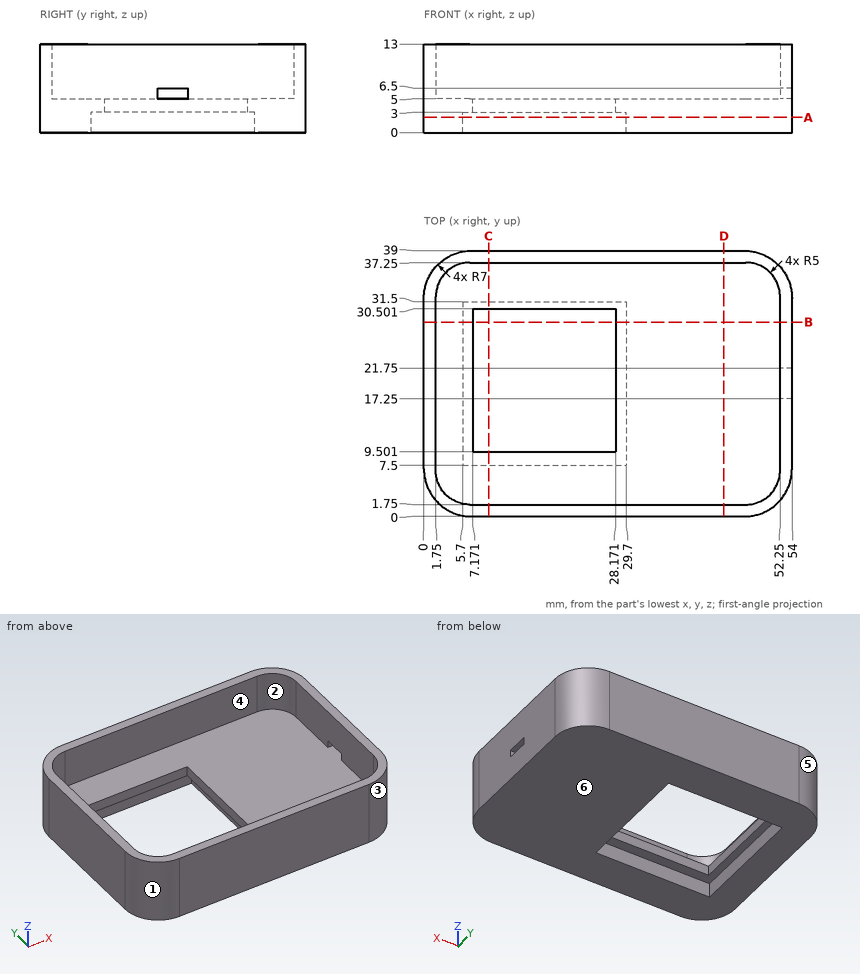
Input: dimensioned drawing with shaded views. Units: mm. Origin: part minimum x, y, z. A direction names the side the tool comes from. Coordinates: 2 decimals unless noted, no trailing zeros. Loops run counter-clockwise (first coordinate to the right, second up) from the corner with the lowest first, then second, coordinate; pieces in that order, holes last. Notation, with made-up numbers: M -25.5,5 L 25.5,5 A23 cw 25.5,26 Z; hole C -34.75,36 d3. An arc over 180 degrees is marked long. Put each result on its own line as item: value.
(1) Cut plane A-A on z = 2.25. Return the cut outline in (x, y), then the cut area to 3 significant figures.
Answer sheet:
outline: M 0,7 A7 ccw 7,0 L 47,0 A7 ccw 54,7 L 54,32 A7 ccw 47,39 L 7,39 A7 ccw 0,32 Z; hole M 5.7,7.5 L 29.7,7.5 L 29.7,31.5 L 5.7,31.5 Z
area: 1,490 mm^2
(2) Access query for the marked faces 1 and 2. Directions: +Z, -Z, +X, -X, +Y, -Y. A direction counts if a zero-diameter tool reaches every point of the face in a straight line with its end or side. Return the directions, or none.
Answer sheet:
face 1: +Z, -Z, -X, -Y
face 2: +Z
(3) Draft query along X for the marked faces 3, 4, 5 and 6. Return one class per face: pulls with the +X half, pulls with the -X half, needs draft (parallel to the pull), parting line crosses it, or undercut.
Answer sheet:
face 3: pulls with the +X half
face 4: undercut
face 5: pulls with the -X half
face 6: needs draft
(4) First-contact query: pin 1 (3.5 mm diameter, centred on x = 12.5, z = 1.5, fed in from -Y); pin 2 (4 mm diameter, centred on x = 17, y = 29.5, fed in from +Z); pin 3 (1.6 mm diameter, centred on x = 53, z = 6, fed in from +Y); pin 4 (0.8 mm diameter, centred on x = 53, z = 5.5, fed in from -Y). Flat tips, straight axial feed; report the tip coordinate or a pass-through.
Answer sheet:
pin 1: stops at y = 0
pin 2: stops at z = 5
pin 3: stops at y = 36.69
pin 4: stops at y = 2.8
(5) Cut plane D-D on x = 44. Return the cut outline in (y, z).
Answer sheet:
outline: M 0,0 L 39,0 L 39,13 L 37.25,13 L 37.25,5 L 1.75,5 L 1.75,13 L 0,13 Z
(6) Cut plane C-C on x = 9.5. Return the cut outline in (y, z).
Answer sheet:
outline: M 0,0 L 7.5,0 L 7.5,3 L 9.5,3 L 9.5,5 L 1.75,5 L 1.75,13 L 0,13 Z; M 30.5,3 L 31.5,3 L 31.5,0 L 39,0 L 39,13 L 37.25,13 L 37.25,5 L 30.5,5 Z
(7) Material intervals for probe 1 along X at (y, z) = (31, 7); probe 2 along X at (y, z) = (25.5, 3.5); probe 3 along Y at (x, z) = (33, 12), sorted ascending.
Answer sheet:
probe 1: x = 0 to 1.75, 52.25 to 54
probe 2: x = 0 to 7.17, 28.17 to 54
probe 3: y = 0 to 1.75, 37.25 to 39
(8) Cut plane B-B on y = 28.5. Return the cut outline in (x, z), then the cut area to 3 significant figures.
Answer sheet:
outline: M 0,0 L 5.7,0 L 5.7,3 L 7.17,3 L 7.17,5 L 1.75,5 L 1.75,13 L 0,13 Z; M 28.17,3 L 29.7,3 L 29.7,0 L 54,0 L 54,13 L 52.25,13 L 52.25,5 L 28.17,5 Z
area: 184 mm^2
